Check sheet for the modelled part. Datum: model origin and axes. Units: mm. Face numbers are marked on the shaded views. A direction names the side the tool comes from. Give positions to 0.01 mm unless a question says otherwise; leave off trailing zeros. Write each loop counter-clockwise with the first axis right and the second up, starting at its lowest first coordinate (ties: lowest second). Pieces come first, ordered by that corner, then holes.
from build123d import *

# Parameters (mm, degrees)
F1_DEPTH = 8


with BuildPart() as f1:
    # F0 (on Top) → F1 (new body)
    with BuildSketch(Plane.XY):
        with BuildLine():
            Line((3.5, 0), (0, 0))
            Line((0, 0), (0, -50))
            Line((0, -50), (29.948091, -50))
            Line((29.948091, -50), (29.948091, 0))
            Line((29.948091, 0), (26.448091, 0))
            ThreePointArc((26.448091, 0), (24.397482, -0.84939), (23.548091, -2.9))
            Line((23.548091, -2.9), (23.548091, -10.99484))
            ThreePointArc((23.548091, -10.99484), (22.31569, -13.493903), (19.582812, -14.037506))
            Line((19.582812, -14.037506), (15.614405, -12.974175))
            ThreePointArc((15.614405, -12.974175), (13.773002, -11.624002), (13.32754, -9.384517))
            Line((13.32754, -9.384517), (16.647826, 9.44576))
            ThreePointArc((16.647826, 9.44576), (16.223577, 11.578604), (14.46986, 12.864482))
            Line((14.46986, 12.864482), (10.276457, 13.988101))
            ThreePointArc((10.276457, 13.988101), (7.673716, 13.470384), (6.5, 11.090324))
            Line((6.5, 11.090324), (6.5, 3))
            ThreePointArc((6.5, 3), (5.62132, 0.87868), (3.5, 0))
        make_face()
    extrude(amount=F1_DEPTH)


solid = f1.part
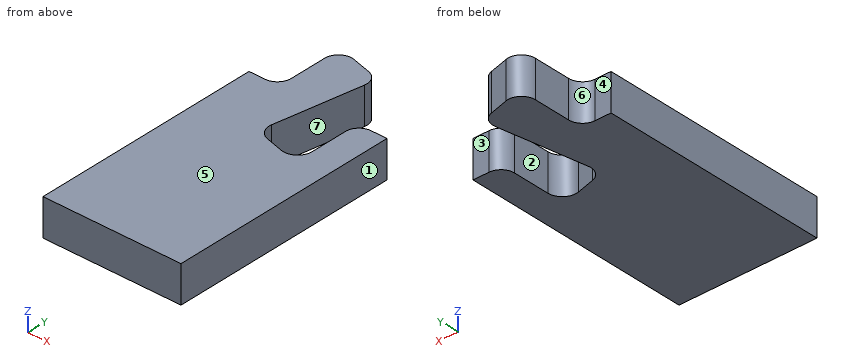
1) Sectioned sample at A-A on z = 1. Record the boundary of the cut face in (x, y).
2) Gauge pin test, flat ends, axial feed: pin 1 (3 mm diameter, centred on x = 29, z = 4.5, fed in from +Y); pin 2 (4 mm diameter, centred on y = 5.5, z = 3.5, fed in from +X). Record the tip position at first contact, or that the pin passes through.
3) Draft check along X on the marked faces 5, 6 and 7. Enter one of: +X half, -X half, draft (parallel to the pull), parting line (faces both ways), or undercut.
4) Sectioned sample at C-C on y = 6. Record the boundary of the cut face in (x, z).
5) Scan lines: L1, parallel to X at y = -11, z = 5.25; L2, parallel to Y at x = 8.75, z = 1.25; L3, parallel to X at y = -3.5, z = 2.25. Record each from-to range of solid material in increasing order.
6) Access from +Z, -Z, +X, -X, +Y, -Y to the whole of each face (thin tool, end or side, straight path). Record for the marked faces 1, 2, 3 and 4.
7) Sectioned sample at B-B on x = 17.75. Record the boundary of the cut face in (y, z), then the cut area to 3 significant figures.
Answers below:
1. outline: (0, -50) - (29.95, -50) - (29.95, 0) - (26.45, 0) arc R2.9 ccw to (23.55, -2.9) - (23.55, -10.99) arc R3.15 cw to (19.58, -14.04) - (15.61, -12.97) arc R3.15 cw to (13.33, -9.38) - (16.65, 9.45) arc R3 ccw to (14.47, 12.86) - (10.28, 13.99) arc R3 ccw to (6.5, 11.09) - (6.5, 3) arc R3 cw to (3.5, 0) - (0, 0) - close
2. pin 1: stops at y = 0
2. pin 2: stops at x = 16.3
3. face 5: draft
3. face 6: -X half
3. face 7: undercut
4. outline: (6.5, 0) - (16.04, 0) - (16.04, 8) - (6.5, 8) - close
5. L1: x = 0 to 13.47, 23.55 to 29.95
5. L2: y = -50 to 14
5. L3: x = 0 to 14.37, 23.55 to 29.95
6. face 1: +Z, -Z, +X, +Y, -Y
6. face 2: +Z, -Z, +Y
6. face 3: +Z, -Z, +X, +Y
6. face 4: +Z, -Z, -X, +Y
7. outline: (-50, 0) - (-13.55, 0) - (-13.55, 8) - (-50, 8) - close
7. area: 292 mm2
